For this review, take the finished solid that the model builds, in its own axes (mm). Face numbers are marked on the shaded views. Coordinates: 2 decimals unless noted, no trailing zeros. Write each loop counter-clockwise with the first axis right and the second up, starting at its lowest first coordinate (ties: lowest second). Pieces come first, ordered by that corner, then holes.
1) Insertion check: P1, Ø4, axis at x = 3, z = -54.5, coming from the +Y side; P2, Ø6, axis at x = -47, z = 41.5, coming from the -Y side; P3, Ø2.5, axis at y = 5.5, z = -3, coming from the +X side; P4, Ø2.5, axis at x = 24.5, y = 6.5, coming from the +Z side. Each pin has a flat end and moves straight along its axis. Give the tip position at first contact, or say it passes through.
2) Mouldability with a two-part tool opening along Z and no side actions: class the marked faces 1 and 2 as pulls with the +Z half, pulls with the -Z half, needs draft (parallel to the pull), parting line crosses it, or undercut.
3) We need section B-B on x = 63.75. Write out the cut boundary in (y, z), then the cut area to 3 significant figures.
4) We need section D-D on x = 30.5. Write out the cut boundary in (y, z), then the cut area to 3 significant figures.
5) We need section C-C on z = -26. Write out the cut boundary in (x, y).
6) We need section A-A on y = -23.5. Write out the cut boundary in (x, z).
7) To check wall thickness, follow line 1 along X through (y, z) = (-3.8, 63.75); line 2 along X through (y, z) = (4.5, -63.75); line 3 along Z through (x, y) = (-63, 2). State the ranges of each line that lie inside material, in increasing order.
from build123d import *

# Parameters (mm, degrees)
SKETCH1_W           = 150
SKETCH1_H           = 150
BOSS_EXTRUDE1_DEPTH = 7.5
BOSS_EXTRUDE2_DEPTH = 114.3
FILLET1_R           = 3
SKETCH3_W           = 20.043778543
SKETCH3_H           = 150
SKETCH3_W_2         = 20
BOSS_EXTRUDE3_DEPTH = 4
SKETCH5_W           = 81
SKETCH5_H           = 102
CUT_EXTRUDE1_DEPTH  = 3
CUT_EXTRUDE3_REACH  = 163.509
SKETCH7_R           = 1.225
BOSS_EXTRUDE4_DEPTH = 3
SKETCH8_R           = 3.5
CUT_EXTRUDE4_DEPTH  = 7.5
SKETCH9_R           = 5
SKETCH9_R_2         = 3.5
BOSS_EXTRUDE5_DEPTH = 6
SKETCH10_R          = 8.5
CUT_EXTRUDE5_DEPTH  = 3


with BuildPart() as part:
    # Sketch1 → Boss-Extrude1 (new body)
    with BuildSketch(Plane(origin=(0, 0, 0), x_dir=(1, 0, 0), z_dir=(0, 1, 0))):
        Rectangle(SKETCH1_W, SKETCH1_H)
    extrude(amount=BOSS_EXTRUDE1_DEPTH)

    # Sketch2 → Boss-Extrude2 (add)
    with BuildSketch(Plane.XZ):
        Polygon((-75, 75), (-55, 75), (-55, 70), (-70, 70), (-70, 55), (-75, 55), align=None)
        Polygon((75, 75), (54.956221457, 75), (54.956221457, 70), (69.950175757, 70), (69.950175757, 55), (75, 55), align=None)
        Polygon((-75, -75), (-55, -75), (-55, -69.976562657), (-70, -69.976562657), (-70, -55.000720359), (-75, -55.000720359), align=None)
        Polygon((75, -75), (54.956221457, -75), (54.956221457, -69.976562657), (69.950175757, -69.976562657), (69.950175757, -55.000720359), (75, -55.000720359), align=None)
    extrude(amount=BOSS_EXTRUDE2_DEPTH)

    # Fillet1
    fillet1_edges = [part.edges().sort_by_distance(p)[0] for p in [
        (-75, 7.5, 0),
        (0, 7.5, 75),
        (75, 7.5, 0),
        (0, 7.5, -75),
    ]]
    fillet(fillet1_edges, radius=FILLET1_R)

    # Sketch3 → Boss-Extrude3 (add)
    with BuildSketch(Plane.XZ.offset(114.3)):
        with Locations((64.978110728, 0)):
            Rectangle(SKETCH3_W, SKETCH3_H)
        with Locations((-65, 0)):
            Rectangle(SKETCH3_W_2, SKETCH3_H)
    extrude(amount=-BOSS_EXTRUDE3_DEPTH)

    # Sketch5 → Cut-Extrude1 (cut)
    with BuildSketch(Plane(origin=(0, 7.5, 0), x_dir=(1, 0, 0), z_dir=(0, 1, 0))):
        Rectangle(SKETCH5_W, SKETCH5_H)
    extrude(amount=-CUT_EXTRUDE1_DEPTH, mode=Mode.SUBTRACT)

    # Sketch6 → Cut-Extrude3 (cut, up to next)
    with BuildSketch(Plane(origin=(0, 7.5, 0), x_dir=(1, 0, 0), z_dir=(0, 1, 0)), mode=Mode.PRIVATE) as cut_extrude3_sk1:
        with BuildLine():
            Line((-50.674102898, 35.299678475), (-50.674102898, -35.299678475))
            ThreePointArc((-50.674102898, -35.299678475), (-56.25, -40.875575577), (-61.825897102, -35.299678475))
            Line((-61.825897102, -35.299678475), (-61.825897102, 35.299678475))
            ThreePointArc((-61.825897102, 35.299678475), (-56.25, 40.875575577), (-50.674102898, 35.299678475))
        make_face()
    cut_extrude3_tool1 = extrude(cut_extrude3_sk1.sketch, amount=-CUT_EXTRUDE3_REACH, mode=Mode.PRIVATE) & part.part
    # Sketch6 → Cut-Extrude3 (cut, up to next)
    with BuildSketch(Plane(origin=(0, 7.5, 0), x_dir=(1, 0, 0), z_dir=(0, 1, 0)), mode=Mode.PRIVATE) as cut_extrude3_sk2:
        with BuildLine():
            Line((61.3258971, 35.299678475), (61.3258971, -35.299678475))
            ThreePointArc((61.3258971, -35.299678475), (56.25, -40.375575575), (51.1741029, -35.299678475))
            Line((51.1741029, -35.299678475), (51.1741029, 35.299678475))
            ThreePointArc((51.1741029, 35.299678475), (56.25, 40.375575575), (61.3258971, 35.299678475))
        make_face()
    cut_extrude3_tool2 = extrude(cut_extrude3_sk2.sketch, amount=-CUT_EXTRUDE3_REACH, mode=Mode.PRIVATE) & part.part
    add(cut_extrude3_tool1.solids().sort_by_distance((-56.25, 7.5, 0))[0], mode=Mode.SUBTRACT)
    add(cut_extrude3_tool2.solids().sort_by_distance((56.25, 7.5, 0))[0], mode=Mode.SUBTRACT)

    # Sketch7 → Boss-Extrude4 (add)
    with BuildSketch(Plane(origin=(0, 4.5, 0), x_dir=(1, 0, 0), z_dir=(0, 1, 0))):
        with Locations(Location((35.5, 46, 0), (0, 0, 270))):
            Circle(SKETCH7_R)
        with Locations(Location((-22.5, 46, 0), (0, 0, 270))):
            Circle(SKETCH7_R)
        with Locations(Location((-22.5, -40, 0), (0, 0, 270))):
            Circle(SKETCH7_R)
        with Locations(Location((35.5, -40, 0), (0, 0, 270))):
            Circle(SKETCH7_R)
    extrude(amount=BOSS_EXTRUDE4_DEPTH)

    # Sketch8 → Cut-Extrude4 (cut)
    with BuildSketch(Plane(origin=(0, 7.5, 0), x_dir=(1, 0, 0), z_dir=(0, 1, 0))):
        with Locations(Location((-63.75, -63.75, 0), (0, 0, 270))):
            Circle(SKETCH8_R)
        with Locations(Location((63.75, -63.75, 0), (0, 0, 270))):
            Circle(SKETCH8_R)
        with Locations(Location((-63.75, 63.75, 0), (0, 0, 270))):
            Circle(SKETCH8_R)
        with Locations(Location((63.75, 63.75, 0), (0, 0, 270))):
            Circle(SKETCH8_R)
    extrude(amount=-CUT_EXTRUDE4_DEPTH, mode=Mode.SUBTRACT)

    # Sketch9 → Boss-Extrude5 (add)
    # profile 1 of 4: a face of its own
    with BuildSketch(Plane.XZ):
        with Locations(Location((-63.75, 63.75, 0), (0, 0, 90))):
            Circle(SKETCH9_R)
        with Locations(Location((-63.75, 63.75, 0), (0, 0, 90))):
            Circle(SKETCH9_R_2, mode=Mode.SUBTRACT)
    # profile 2 of 4: a face of its own
    with BuildSketch(Plane.XZ):
        with Locations(Location((63.75, 63.75, 0), (0, 0, 90))):
            Circle(SKETCH9_R)
        with Locations(Location((63.75, 63.75, 0), (0, 0, 90))):
            Circle(SKETCH9_R_2, mode=Mode.SUBTRACT)
    # profile 3 of 4: a face of its own
    with BuildSketch(Plane.XZ):
        with Locations(Location((63.75, -63.75, 0), (0, 0, 90))):
            Circle(SKETCH9_R)
        with Locations(Location((63.75, -63.75, 0), (0, 0, 90))):
            Circle(SKETCH9_R_2, mode=Mode.SUBTRACT)
    # profile 4 of 4: a face of its own
    with BuildSketch(Plane.XZ):
        with Locations(Location((-63.75, -63.75, 0), (0, 0, 90))):
            Circle(SKETCH9_R)
        with Locations(Location((-63.75, -63.75, 0), (0, 0, 90))):
            Circle(SKETCH9_R_2, mode=Mode.SUBTRACT)
    extrude(amount=BOSS_EXTRUDE5_DEPTH)

    # Sketch10 → Cut-Extrude5 (cut)
    with BuildSketch(Plane(origin=(0, 7.5, 0), x_dir=(1, 0, 0), z_dir=(0, 1, 0))):
        with Locations((0, 51)):
            Circle(SKETCH10_R)
        with Locations((0, -51)):
            Circle(SKETCH10_R)
    extrude(amount=-CUT_EXTRUDE5_DEPTH, mode=Mode.SUBTRACT)


solid = part.part
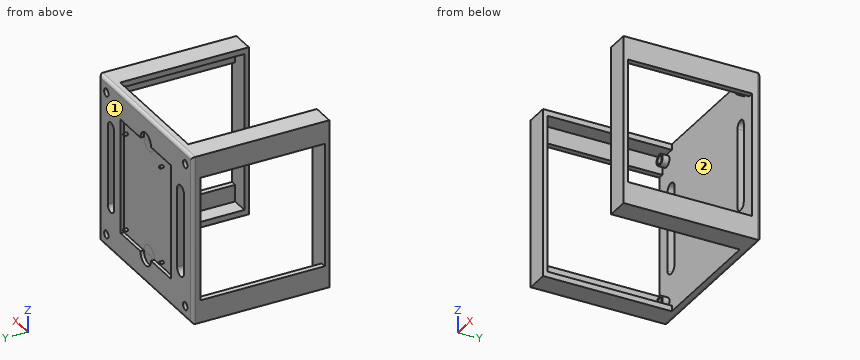
Result:
1. P1: stops at y = 4.5
1. P2: stops at y = 0
1. P3: stops at x = 75
1. P4: stops at z = 74.9
2. face 1: needs draft
2. face 2: undercut
3. outline: (-114.3, -75) - (4.5, -75) arc R3 ccw to (7.5, -72) - (7.5, -67.25) - (-6, -67.25) - (-6, -68.75) - (0, -68.75) - (0, -69.98) - (-110.3, -69.98) - (-110.3, 70) - (0, 70) - (0, 68.75) - (-6, 68.75) - (-6, 67.25) - (7.5, 67.25) - (7.5, 72) arc R3 ccw to (4.5, 75) - (-114.3, 75) - close; (-6, -60.25) - (7.5, -60.25) - (7.5, 60.25) - (-6, 60.25) - (-6, 58.75) - (0, 58.75) - (0, -58.75) - (-6, -58.75) - close
3. area: 2,760 mm2
4. outline: (0, -75) - (4.5, -75) arc R3 ccw to (7.5, -72) - (7.5, -51) - (4.5, -51) - (4.5, 51) - (7.5, 51) - (7.5, 72) arc R3 ccw to (4.5, 75) - (0, 75) - close
4. area: 815 mm2
5. outline: (-75, -114.3) - (-55, -114.3) - (-55, -110.3) - (-75, -110.3) - close; (-75, 0) - (-61.83, 0) - (-61.83, 7.5) - (-72, 7.5) arc R3 ccw to (-75, 4.5) - close; (-50.67, 0) - (51.17, 0) - (51.17, 7.5) - (40.5, 7.5) - (40.5, 4.5) - (-40.5, 4.5) - (-40.5, 7.5) - (-50.67, 7.5) - close; (54.96, -114.3) - (75, -114.3) - (75, -110.3) - (54.96, -110.3) - close; (61.33, 0) - (75, 0) - (75, 4.5) arc R3 ccw to (72, 7.5) - (61.33, 7.5) - close
6. outline: (-75, -75) - (-55, -75) - (-55, -69.98) - (-70, -69.98) - (-70, -55) - (-75, -55) - close; (-75, 55) - (-70, 55) - (-70, 70) - (-55, 70) - (-55, 75) - (-75, 75) - close; (54.96, -75) - (75, -75) - (75, -55) - (69.95, -55) - (69.95, -69.98) - (54.96, -69.98) - close; (54.96, 70) - (69.95, 70) - (69.95, 55) - (75, 55) - (75, 75) - (54.96, 75) - close
7. line 1: x = -75 to -70, -68.75 to -67.25, -60.25 to -58.75, 58.75 to 60.25, 67.25 to 68.75, 69.95 to 75
7. line 2: x = -75 to -67.25, -60.25 to 60.25, 67.25 to 75
7. line 3: z = -75 to -67.17, -60.33 to 60.33, 67.17 to 75
